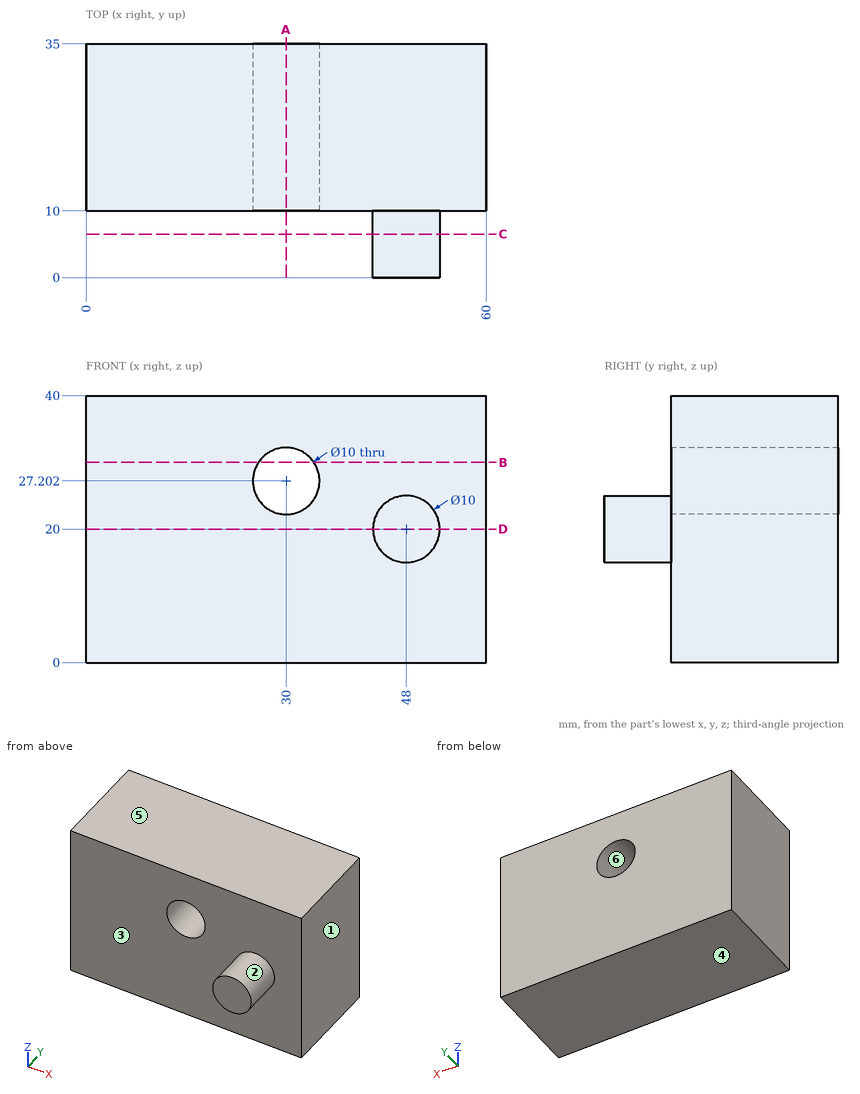
Verification items for this drawing (mm, ordinates from the low corner). A direction names the side the tool comes from. Coordinates: 2 decimals unless noted, no trailing zeros. Order: outer loops, then holes, each group sorted by start corner. A loop starts at its lowest first (then second) coordinate and runs counter-clockwise, first axis right, second up. Notation, with made-up numbers: M 54,40 L 96,40 A25 ccw 96,58 Z; hole C -25.75,29 d4. An arc over 180 degrees is marked long. Write each question's results on one line, items separated by ' | '.
1) Scan lines: line 1 along Z through (x, y) = (30, 18); line 2 along Y through (x, z) = (4, 24.5); line 3 along X through (y, z) = (31, 30.5). Record each from-to range of solid material in increasing order. Write a range as [from, to].
Solved:
line 1: z = [0, 22.2], [32.2, 40] | line 2: y = [10, 35] | line 3: x = [0, 26.24], [33.76, 60]
2) Gauge pin test, flat end, axial feed: pin 1 Ø5 at (x, z) = (43.5, 35.5) entering from -Y. Record the tip position at first contact, or that the pin passes through.
Solved:
pin 1: stops at y = 10
3) Section check C-C on y = 6.5. Record the cut outline in (x, z).
Solved:
outline: C 48,20 d10
4) Section check B-B on z = 30. Record the cut outline in (x, y).
Solved:
outline: M 0,10 L 25.86,10 L 25.86,35 L 0,35 Z; M 34.14,10 L 60,10 L 60,35 L 34.14,35 Z
5) Release check for a two-part mould opening along Z. For the marked faces 3, 4, 5 and 6 record: pulls with the +Z half, pulls with the -Z half, needs draft (parallel to the pull), parting line crosses it, or undercut.
Solved:
face 3: needs draft | face 4: pulls with the -Z half | face 5: pulls with the +Z half | face 6: undercut
6) Section check A-A on x = 30. Record the cut outline in (y, z).
Solved:
outline: M 10,0 L 35,0 L 35,22.2 L 10,22.2 Z; M 10,32.2 L 35,32.2 L 35,40 L 10,40 Z
7) Section check D-D on z = 20. Record the cut outline in (x, y), plus the area to 3 significant figures.
Solved:
outline: M 0,10 L 43,10 L 43,0 L 53,0 L 53,10 L 60,10 L 60,35 L 0,35 Z | area: 1,600 mm²
8) Access from +Z, -Z, +X, -X, +Y, -Y to the whole of each face (thin tool, end or side, straight path). Record for the marked faces 1 and 2.
Solved:
face 1: +Z, -Z, +X, +Y, -Y | face 2: -Y
